Print and shaded views of the part. All mm, measured from the part's lowest x, y and z. A direction names the side the tool comes from. Coordinates: 2 decimals unless noted, no trailing zeros. Loops run counter-clockwise (first coordinate to the right, second up) from the corner with the lowest first, then second, coordinate; pieces in that order, holes last. Notation, with made-up numbers: M -37.5,35.25 L -18.5,35.25 A15 ccw -18.5,58.25 Z; hole C 57,51 d1. An arc over 180 degrees is marked long. Answer as a JSON object with one key per item and string values. Group by question number.
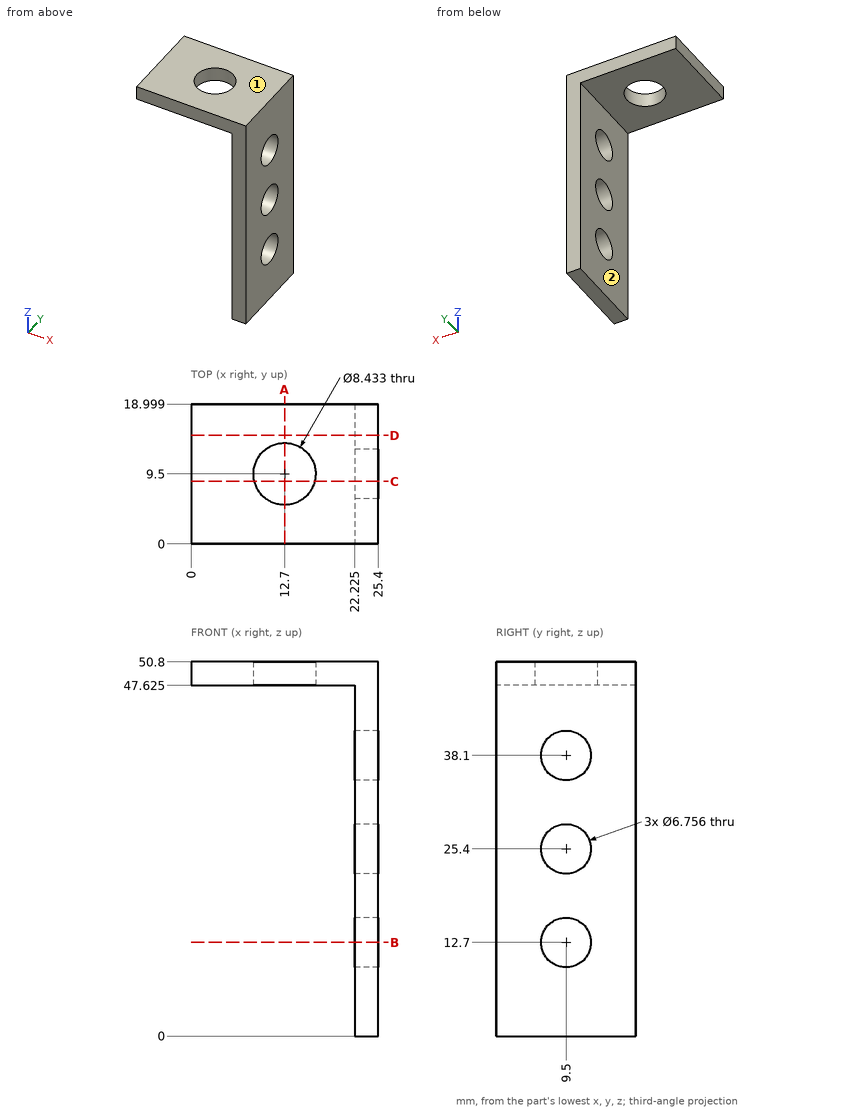
Item 1: Drill centre lines: L1, parallel to Y at x = 12.7, z = 48.3; L2, parallel to Y at x = 24.1, z = 25.4; L3, parallel to X at y = 14, z = 39 (1 decimal). Where is each one in solid material? Low to high. Write a range as from..to.
Item 2: Slice it at D-D, the plane y = 14.75. Write the cut outline in (x, z) (1 decimal), then the cut area to 3 significant figures.
Item 3: Pin check, flat tip, straight feed: pin 1 (2 mm diameter, centred on y = 2.5, z = 25.5, fed in from -X) (3 decimals). Stop position of the tip, or through.
Item 4: Tool access for the marked faces 1 and 2: list every direction of +Z, -Z, +X, -X, +Y, -Y with a clear straight run to the whole face (end or side of a thin tool).
Item 5: Slice it at B-B, the plane z = 12.7. Write the cut outline in (x, y) (1 decimal).
Item 6: Slice it at A-A, the plane x = 12.7. Write the cut outline in (y, z) (1 decimal).
Item 7: Slice it at C-C, the plane y = 8.5. Write the cut outline in (x, z) (1 decimal), then the cut area to 3 significant figures.
Computed:
{
 "1": {"L1": "0..5.28, 13.72..19", "L2": "0..6.12, 12.88..19", "L3": "22.2..25.4"},
 "2": {"outline": "M 0,47.6 L 22.2,47.6 L 22.2,0 L 25.4,0 L 25.4,50.8 L 0,50.8 Z", "area": "232 mm2"},
 "3": {"pin 1": "x = 22.225"},
 "4": {"face 1": "+Z, +X, -X, +Y, -Y", "face 2": "-Z, -X, +Y, -Y"},
 "5": {"outline": "M 22.2,0 L 25.4,0 L 25.4,6.1 L 22.2,6.1 Z; M 22.2,12.9 L 25.4,12.9 L 25.4,19 L 22.2,19 Z"},
 "6": {"outline": "M 0,47.6 L 5.3,47.6 L 5.3,50.8 L 0,50.8 Z; M 13.7,47.6 L 19,47.6 L 19,50.8 L 13.7,50.8 Z"},
 "7": {"outline": "M 0,47.6 L 8.6,47.6 L 8.6,50.8 L 0,50.8 Z; M 16.8,47.6 L 22.2,47.6 L 22.2,41.3 L 25.4,41.3 L 25.4,50.8 L 16.8,50.8 Z; M 22.2,0 L 25.4,0 L 25.4,9.5 L 22.2,9.5 Z; M 22.2,15.9 L 25.4,15.9 L 25.4,22.2 L 22.2,22.2 Z; M 22.2,28.6 L 25.4,28.6 L 25.4,34.9 L 22.2,34.9 Z", "area": "144 mm2"}
}
